from build123d import *

# Parameters (mm, degrees)
F0_W      = 38.1
F0_H      = 31.75
F1_DEPTH  = 25.4
F1_FACE_W = 25.4
F1_FACE_H = 31.75
F3_DEPTH  = 25.4


with BuildPart() as f1:
    # F0 (on Front) → F1 (new body)
    with BuildSketch(Plane.XZ):
        with Locations((23.058977, 25.241072)):
            Rectangle(F0_W, F0_H)
    extrude(amount=F1_DEPTH)

    # F2 (on Right) + F1_face (on face) → F3 (cut)
    with BuildSketch(Plane.YZ):
        Polygon((-25.473946, 41.330271), (-25.473946, 15.930271), (-6.423946, 41.330271), align=None)
    with BuildSketch(Plane(origin=(42.108977, -12.7, 25.241072), x_dir=(0, 1, 0), z_dir=(1, 0, 0))):
        Rectangle(F1_FACE_W, F1_FACE_H)
    extrude(amount=F3_DEPTH, mode=Mode.SUBTRACT)


solid = f1.part
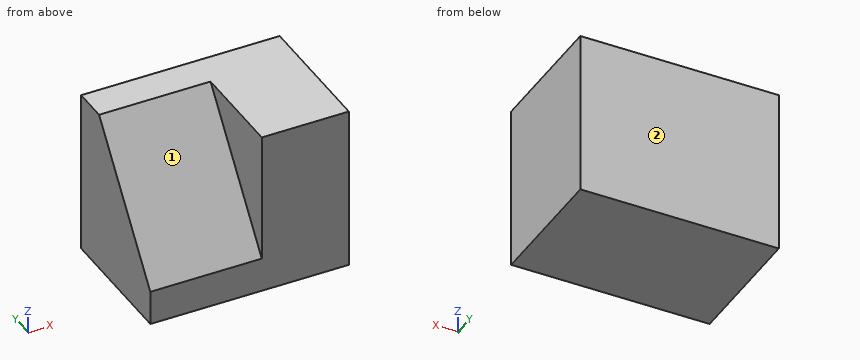
Source: CAD feature listing. Evaluate the final solid. Frame: model axes, mm. Face numbers are marked on the shaded views. A direction names the side the tool comes from. Round coordinates to 2 decimals unless told otherwise and drop trailing zeros. Order: outer loops, then holes, each group sorted by start corner. A loop starts at its lowest first (then second) coordinate and runs counter-clockwise, first axis right, second up. Notation, with made-up numbers: (-8.5, 2) - (32.5, 2) arc R33 cw to (32.5, 38) - close; hole circle Ø3 at (16, -5.75). An arc over 180 degrees is marked (long way). Use a Markdown table: item, result. Add a question column.
1. Section query B-B (z = 39). Return the cut outline in (x, y), then the cut area to 3 significant figures.
2. Section query C-C (y = -15.25). Return the cut outline in (x, z), then the cut area to 3 significant figures.
3. Set-up query: the marked faces 1 and 2. Return all of +Z, -Z, +X, -X, +Y, -Y with unobstructed straight access to the full face (end or side cutting, diameter ignored); none if empty.
4. Section query A-A (x = 23). Return the cut outline in (y, z).
5. First-contact query: pin 1 (12 mm diameter, centred on x = 19, z = 22.5, fed in from -Y). Flat tip, straight axial feed; report the tip coordinate or a pass-through.
6. Line query: probe 1 along X at (y, z) = (-21, 36.5); probe 2 along Z at (x, y) = (20, -24); probe 3 along Z at (x, y) = (7.5, -17). Output: solid intervals per line, ascending.
Derived:
| question | item | result |
|---|---|---|
| 1 | outline | (4.01, -8.17) - (25.4, -8.17) - (25.4, -25.4) - (42.11, -25.4) - (42.11, 0) - (4.01, 0) - close |
| 1 | area | 599 mm2 |
| 2 | outline | (4.01, 9.37) - (42.11, 9.37) - (42.11, 41.12) - (25.4, 41.12) - (25.4, 29.56) - (4.01, 29.56) - close |
| 2 | area | 963 mm2 |
| 3 | face 1 | +Z, -X, -Y |
| 3 | face 2 | +Z, -Z, +X, -X, +Y |
| 4 | outline | (-25.4, 9.37) - (0, 9.37) - (0, 41.12) - (-6.58, 41.12) - (-25.4, 16.03) - close |
| 5 | pin 1 | y = -25.05 |
| 6 | probe 1 | 25.4 to 42.11 |
| 6 | probe 2 | 9.37 to 17.9 |
| 6 | probe 3 | 9.37 to 27.23 |
